Verification items for the finished model (mm, model axes). Face numbers are marked on the shaded views. A direction names the side the tool comes from. Coordinates: 2 decimals unless noted, no trailing zeros. Order: outer loops, then holes, each group sorted by start corner. A loop starts at its lowest first (then second) coordinate and runs counter-clockwise, first axis right, second up. Notation, with made-up numbers: M 69.5,9.5 L 92.5,9.5 A11 cw 92.5,13.5 Z; hole C -11,-7 d9. An arc over 180 degrees is marked long. Return JSON: item names as keys, results as strings.
```python
from build123d import *

# Parameters (mm, degrees)
SKETCH2_R          = 8
BODY_EXTRUDE_DEPTH = 5
BODY_FILLET_A_R    = 1.5875
BODY_FILLET_B_R    = 1.5875
CHAMFER2_SIZE      = 1.5875
ID_CHAMFER_SIZE    = 0.381
SKETCH3_R          = 3.571875
HOLE_CUT_DEPTH     = 37.746054285


with BuildPart() as part:
    # Sketch2 → Body Extrude (new, symmetric)
    with BuildSketch(Plane.XY):
        with BuildLine():
            Line((-28.5, 0), (-28.5, 6.35))
            Line((-28.5, 6.35), (-14.7, 6.35))
            Line((-14.7, 6.35), (-14.7, 14.3))
            ThreePointArc((-14.7, 14.3), (0, 29), (14.7, 14.3))
            Line((14.7, 14.3), (14.7, 6.35))
            Line((14.7, 6.35), (28.5, 6.35))
            Line((28.5, 6.35), (28.5, 0))
            Line((28.5, 0), (-28.5, 0))
        make_face()
        with Locations((0, 14.3)):
            Circle(SKETCH2_R, mode=Mode.SUBTRACT)
    extrude(amount=BODY_EXTRUDE_DEPTH, both=True)

    # Body Fillet A
    body_fillet_a_edges = [part.edges().sort_by_distance(p)[0] for p in [
        (14.7, 10.325, 5),
        (0, 29, 5),
        (-14.7, 10.325, 5),
        (-14.7, 10.325, -5),
        (0, 29, -5),
        (14.7, 10.325, -5),
    ]]
    fillet(body_fillet_a_edges, radius=BODY_FILLET_A_R)

    # Body Fillet B
    # the kernel refuses this fillet: 1.5875 mm, written as the material it adds along each edge
    with BuildSketch(Plane(origin=(-14.7, 6.35, 3.4125), x_dir=(0, 1, 0), z_dir=(0, 0, -1))) as body_fillet_b_piece_1:
        with BuildLine():
            CenterArc((BODY_FILLET_B_R, -BODY_FILLET_B_R), BODY_FILLET_B_R, 90, 90)
            Line((0, -BODY_FILLET_B_R), (0, 0))
            Line((0, 0), (BODY_FILLET_B_R, 0))
        make_face()
    extrude(amount=6.825)
    with BuildSketch(Plane(origin=(14.7, 6.35, 3.4125), x_dir=(0, 1, 0), z_dir=(0, 0, -1))) as body_fillet_b_piece_2:
        with BuildLine():
            CenterArc((BODY_FILLET_B_R, BODY_FILLET_B_R), BODY_FILLET_B_R, 180, 90)
            Line((0, BODY_FILLET_B_R), (0, 0))
            Line((0, 0), (BODY_FILLET_B_R, 0))
        make_face()
    extrude(amount=6.825)
    with BuildSketch(Plane(origin=(-13.1125, 6.35, -3.4125), x_dir=(-1, 0, 0), z_dir=(0, 0, 1))) as body_fillet_b_piece_3_section:
        with BuildLine():
            CenterArc((1.5875 + BODY_FILLET_B_R, -BODY_FILLET_B_R), BODY_FILLET_B_R, 90, 90)
            Line((1.5875 + BODY_FILLET_B_R, 0), (1.5875, 0))
            Line((1.5875, 0), (1.5875, -BODY_FILLET_B_R))
        make_face()
    body_fillet_b_piece_3 = revolve(axis=Axis((-13.1125, 6.35, -3.4125), (0, -1, 0)), revolution_arc=233.296989237, mode=Mode.PRIVATE)
    body_fillet_b_piece_3 = split(body_fillet_b_piece_3, bisect_by=Plane(origin=(-14.303028138, 6.844709666, -5), z_dir=(0, 0, 1)), keep=Keep.TOP, mode=Mode.PRIVATE)
    add(body_fillet_b_piece_3)
    with BuildSketch(Plane(origin=(13.1125, 6.35, 3.4125), x_dir=(-0.597667277632828, 0, -0.8017442392976478), z_dir=(0.8017442392976478, 0, -0.597667277632828))) as body_fillet_b_piece_4_section:
        with BuildLine():
            CenterArc((1.5875 + BODY_FILLET_B_R, BODY_FILLET_B_R), BODY_FILLET_B_R, 180, 90)
            Line((1.5875, BODY_FILLET_B_R), (1.5875, 0))
            Line((1.5875, 0), (1.5875 + BODY_FILLET_B_R, 0))
        make_face()
    body_fillet_b_piece_4 = revolve(axis=Axis((13.1125, 6.35, 3.4125), (0, 1, 0)), revolution_arc=233.296989237, mode=Mode.PRIVATE)
    body_fillet_b_piece_4 = split(body_fillet_b_piece_4, bisect_by=Plane(origin=(14.303027956, 6.844710216, 5), z_dir=(0, 0, -1)), keep=Keep.TOP, mode=Mode.PRIVATE)
    add(body_fillet_b_piece_4)
    with BuildSketch(Plane(origin=(13.1125, 6.35, -3.4125), x_dir=(1, 0, 0), z_dir=(0, 0, 1))) as body_fillet_b_piece_5_section:
        with BuildLine():
            CenterArc((1.5875 + BODY_FILLET_B_R, BODY_FILLET_B_R), BODY_FILLET_B_R, 180, 90)
            Line((1.5875 + BODY_FILLET_B_R, 0), (1.5875, 0))
            Line((1.5875, 0), (1.5875, BODY_FILLET_B_R))
        make_face()
    body_fillet_b_piece_5 = revolve(axis=Axis((13.1125, 6.35, -3.4125), (0, 1, 0)), revolution_arc=233.296989237, mode=Mode.PRIVATE)
    body_fillet_b_piece_5 = split(body_fillet_b_piece_5, bisect_by=Plane(origin=(14.303027986, 6.84471004, -5), z_dir=(0, 0, 1)), keep=Keep.TOP, mode=Mode.PRIVATE)
    add(body_fillet_b_piece_5)
    with BuildSketch(Plane(origin=(-13.1125, 6.35, 3.4125), x_dir=(0.597667277632828, 0, -0.8017442392976478), z_dir=(-0.8017442392976478, 0, -0.597667277632828))) as body_fillet_b_piece_6_section:
        with BuildLine():
            CenterArc((1.5875 + BODY_FILLET_B_R, -BODY_FILLET_B_R), BODY_FILLET_B_R, 90, 90)
            Line((1.5875 + BODY_FILLET_B_R, 0), (1.5875, 0))
            Line((1.5875, 0), (1.5875, -BODY_FILLET_B_R))
        make_face()
    body_fillet_b_piece_6 = revolve(axis=Axis((-13.1125, 6.35, 3.4125), (0, -1, 0)), revolution_arc=233.296989237, mode=Mode.PRIVATE)
    body_fillet_b_piece_6 = split(body_fillet_b_piece_6, bisect_by=Plane(origin=(-14.30302807, 6.844709941, 5), z_dir=(0, 0, -1)), keep=Keep.TOP, mode=Mode.PRIVATE)
    add(body_fillet_b_piece_6)

    # Chamfer2
    chamfer2_edges = [part.edges().sort_by_distance(p)[0] for p in [
        (28.5, 3.175, -5),
        (-28.5, 3.175, 5),
        (28.5, 3.175, 5),
        (-28.5, 3.175, -5),
    ]]
    chamfer(chamfer2_edges, length=CHAMFER2_SIZE)

    # ID Chamfer
    id_chamfer_edges = [part.edges().sort_by_distance(p)[0] for p in [
        (-8, 14.3, -5),
        (-8, 14.3, 5),
    ]]
    chamfer(id_chamfer_edges, length=ID_CHAMFER_SIZE)

    # Sketch3 → Hole Cut (cut, through all)
    with BuildSketch(Plane(origin=(0, 6.35, 0), x_dir=(1, 0, 0), z_dir=(0, 1, 0))):
        with Locations(Location((-22, 0, 0), (0, 0, 180))):
            Circle(SKETCH3_R)
        with Locations((22, 0)):
            Circle(SKETCH3_R)
    extrude(amount=-HOLE_CUT_DEPTH, mode=Mode.SUBTRACT)


solid = part.part
```
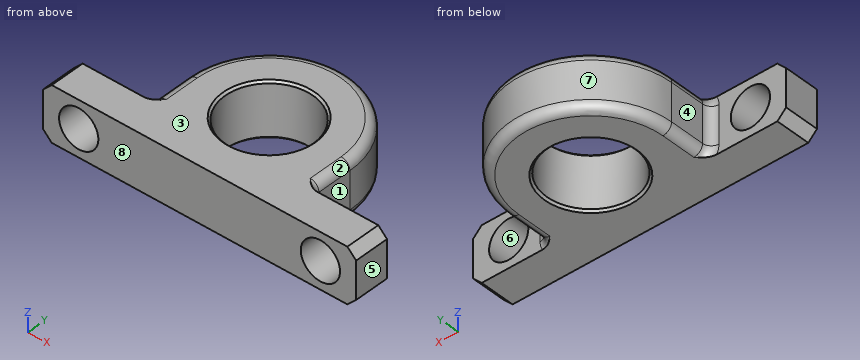
Q1. Cross-section at A-A, the plane x = -22. Record the boundary of the cut face in (y, z).
Values:
{"outline": "M 0,-5 L 6.35,-5 L 6.35,-3.57 L 0,-3.57 Z; M 0,3.57 L 6.35,3.57 L 6.35,5 L 0,5 Z"}
Q2. Tool access check on the marked faces 1, 2, 3, 4 and 5. Record the directions out of +Z, -Z, +X, -X, +Y, -Y that give a thin tool (end or side, any length) a straight path to the whole face; none if there is none.
Values:
{"face 1": "+Z, -Z, +X, +Y", "face 2": "+Z, +X, +Y", "face 3": "+Z, +X, -X, +Y, -Y", "face 4": "+Z, -Z, -X, +Y", "face 5": "+Z, -Z, +X, +Y, -Y"}
Q3. Material ranges on line 1 along Y through (x, z) = (0, -1.75); line 2 along Z through (x, y) = (22, 2.5); line 3 along X through (y, z) = (2.5, -1.5), recorded low to high.
Values:
{"line 1": "0 to 6.3, 22.3 to 29", "line 2": "-5 to -3.57, 3.57 to 5", "line 3": "-28.5 to -25.24, -18.76 to 18.76, 25.24 to 28.5"}
Q4. Draft check along X on the marked faces 6, 7 and 8. Enter one of: pulls with the +X half, pulls with the -X half, needs draft (parallel to the pull), parting line crosses it, or undercut.
Values:
{"face 6": "undercut", "face 7": "parting line crosses it", "face 8": "needs draft"}
Q5. Cross-section at C-C, the plane x = 0. Record the boundary of the cut face in (y, z) (1 decimal), and give its area (3 significant figures).
Values:
{"outline": "M 0,-5 L 5.9,-5 L 6.3,-4.6 L 6.3,4.6 L 5.9,5 L 0,5 Z; M 22.3,-4.6 L 22.7,-5 L 27.4,-5 A1.6 ccw 29,-3.4 L 29,3.4 A1.6 ccw 27.4,5 L 22.7,5 L 22.3,4.6 Z", "area": "129 mm^2"}
Q6. Cross-section at B-B, the plane z = 0. State how many separate pieces and enclosed holes the cut face has, and give its area (3 significant figures).
Values:
{"separate pieces": "3", "enclosed holes": "1", "area": "644 mm^2"}
Q7. Go/stop test with flat-tipped pins: pin 1 (6 mm diameter, centred on y = 24, z = -1.5, fed in from +X); pin 2 (3 mm diameter, centred on y = 22, z = 1.5, fed in from +X); pin 3 (1 mm diameter, centred on y = 8.5, z = 0.5, fed in from -X). Record where each tip stops, or that it passes through.
Values:
{"pin 1": "x = 13.08", "pin 2": "x = 13.33", "pin 3": "x = -14.7"}
